Autodesk Inventor part; units mm, degrees
ref_plane "YZ Plane" through (0, 0, 0) normal (1, 0, 0) x (0, 1, 0)
ref_plane "XZ Plane" through (0, 0, 0) normal (0, 1, 0) x (-1, 0, 0)
ref_plane "XY Plane" through (0, 0, 0) normal (0, 0, 1) x (1, 0, 0)
sketch "Sketch1" plane through (0, 0, 0) normal (0, 0, 1) x (1, 0, 0)
  line L0 (-29.75, -11.25) -> (29.75, -11.25)
  line L1 (29.75, -11.25) -> (29.75, 11.25)
  line L2 (29.75, 11.25) -> (-29.75, 11.25)
  line L3 (-29.75, 11.25) -> (-29.75, -11.25)
  line L4 (-29.75, -11.25) -> (29.75, 11.25) construction
  line L5 (29.75, -11.25) -> (-29.75, 11.25) construction
  point P0 (0, 0)
  dimension "d0" = 59.5
  dimension "d1" = 22.5
extrude "Extrusion1" add sketch "Sketch1" against normal blind 1.6
fillet "Fillet1" radius 1.5 4 edges at (29.75, 11.25, -0.8) (29.75, -11.25, -0.8) (-29.75, 11.25, -0.8) (-29.75, -11.25, -0.8)
sketch "Sketch2" plane through (0, 0, 0) normal (0, 0, 1) x (1, 0, 0)
  circle A0 centre (-2.949, 1.26) radius 4.75
  line L0 (-28.25, -11.25) -> (28.25, -11.25)
  line L1 (-29.75, 9.75) -> (-29.75, -9.75)
  line L2 (-24.199, -4.44) -> (-19.799, -4.44)
  line L3 (-19.799, -4.44) -> (-19.799, -2.04)
  line L4 (-19.799, -2.04) -> (-24.199, -2.04)
  line L5 (-24.199, -2.04) -> (-24.199, -4.44)
  line L6 (-24.199, -4.44) -> (-19.799, -2.04) construction
  line L7 (-19.799, -4.44) -> (-24.199, -2.04) construction
  point P0 (0, 0)
  point P1 (-28.349, -5.24)
  point P2 (-21.999, -3.24)
  dimension "d5" = 9.5
  dimension "d15" = 12.51
  dimension "d16" = 26.801
  dimension "d17" = 6.01
  dimension "d18" = 1.401
  dimension "d19" = 4.4
  dimension "d20" = 2.4
  dimension "d21" = 6.35
  dimension "d22" = 2
extrude "Extrusion2" cut sketch "Sketch2" against normal through all
sketch "Sketch4" plane through (0, 0, 0) normal (0, 0, 1) x (1, 0, 0)
  line L0 (-28.25, -11.25) -> (28.25, -11.25)
  line L1 (-29.75, 9.75) -> (-29.75, -9.75)
  line L2 (6.731, -5.34) -> (22.931, -5.34)
  line L3 (22.931, -5.34) -> (22.931, 2.86)
  line L4 (22.931, 2.86) -> (6.731, 2.86)
  line L5 (6.731, 2.86) -> (6.731, -5.34)
  line L6 (6.731, -5.34) -> (22.931, 2.86) construction
  line L7 (22.931, -5.34) -> (6.731, 2.86) construction
  point P0 (0, 0)
  point P1 (-28.349, -5.24)
  point P2 (14.831, -1.24)
  dimension "d23" = 6.01
  dimension "d24" = 1.401
  dimension "d25" = 16.2
  dimension "d26" = 8.2
  dimension "d28" = 43.18
  dimension "d29" = 0.1
extrude "Extrusion4" cut sketch "Sketch4" against normal through all
sketch "Sketch5" plane through (0, 0, -1.6) normal (0, 0, -1) x (-1, 0, 0)
  line L0 (-29.75, 11.25) -> (29.75, 11.25) construction
  line L1 (29.75, 11.25) -> (29.75, -11.2327) construction
  line L2 (29.75, -11.2327) -> (-29.75, -11.2327) construction
  line L3 (-29.75, -11.2327) -> (-29.75, 11.25) construction
  line L4 (28.25, 11.25) -> (-28.25, 11.25)
  line L5 (-29.75, 9.75) -> (-29.75, -9.75)
  line L6 (29.75, -9.75) -> (29.75, 9.75)
  point P0 (0, 0)
decal "Decal1"
properties part number "rearPlate_PP"
The model under review builds one solid part; all positions refer to its coordinate system, in mm. A direction names the side the tool comes from. Round coordinates to 2 decimals unless told otherwise and drop trailing zeros. Loops run counter-clockwise (first coordinate to the right, second up) from the corner with the lowest first, then second, coordinate; pieces in that order, holes last. Notation, with made-up numbers: (60.5, 27) -> (69.5, 27) arc R28 cw to (69.5, 52) -> close; hole circle Ø9 at (-10.5, 5). An arc over 180 degrees is marked (long way). Answer as a JSON object with one key per item and string values. Group by question number.
1) We need section B-B on x = 20.5. Write out the cut boundary in (y, z), then the cut area to 3 significant figures.
2) We need section D-D on x = -4. Write out the cut boundary in (y, z), then the cut area to 3 significant figures.
3) For pin 1 Ø5.5 at (x, y) = (-2.949, 1.26) entering from +Z, flat-tipped, find the tip position at first contact; note if it passes through.
4) We need section A-A on y = 1.26. Write out the cut boundary in (x, z).
5) We need section C-C on z = -1.1. Write out the cut boundary in (x, y), then the cut area to 3 significant figures.
6) For line 1 (Y direction, x = 19.5, z = -1.05); line 2 (X direction, y = -0.5, z = -0.35); line 3 (X direction, y = 2.75, z = -0.65), list the stretches that pass through material, from the lowest coordinate up. Write a range as [from, to].
7) Mouldability with a two-part tool opening along Y and no side actions: class faces 1 (the face through (-22, -4.44, -1)), 2 (the face through (-29.3, -10.82, -0.81)), 3 (the face through (0, -5, -1.6)) as released by +Y, released by -Y, zero draft, split by the parting line, or undercut.
8) For faces 4 (the face through (-29.75, 0, -1)), 5 (the face through (6.731, -1, -1)), list the 3-axis set-ups (+Z, -Z, +X, -X, +Y, -Y) from which the entire face can be reached by the end or side of a thin tool; tool diameter is ignored.
Result set:
{
 "1": {"outline": "(-11.25, -1.6) -> (-5.34, -1.6) -> (-5.34, 0) -> (-11.25, 0) -> close; (2.86, -1.6) -> (11.25, -1.6) -> (11.25, 0) -> (2.86, 0) -> close", "area": "22.9 mm²"},
 "2": {"outline": "(-11.25, -1.6) -> (-3.37, -1.6) -> (-3.37, 0) -> (-11.25, 0) -> close; (5.89, -1.6) -> (11.25, -1.6) -> (11.25, 0) -> (5.89, 0) -> close", "area": "21.2 mm²"},
 "3": {"pin 1": "through"},
 "4": {"outline": "(-29.75, -1.6) -> (-7.7, -1.6) -> (-7.7, 0) -> (-29.75, 0) -> close; (1.8, -1.6) -> (6.73, -1.6) -> (6.73, 0) -> (1.8, 0) -> close; (22.93, -1.6) -> (29.75, -1.6) -> (29.75, 0) -> (22.93, 0) -> close"},
 "5": {"outline": "(-29.75, -9.75) arc R1.5 ccw to (-28.25, -11.25) -> (28.25, -11.25) arc R1.5 ccw to (29.75, -9.75) -> (29.75, 9.75) arc R1.5 ccw to (28.25, 11.25) -> (-28.25, 11.25) arc R1.5 ccw to (-29.75, 9.75) -> close; hole (-24.2, -4.44) -> (-19.8, -4.44) -> (-19.8, -2.04) -> (-24.2, -2.04) -> close; hole circle Ø9.5 at (-2.95, 1.26); hole (6.73, -5.34) -> (22.93, -5.34) -> (22.93, 2.86) -> (6.73, 2.86) -> close", "area": "1,120 mm²"},
 "6": {"line 1": "[-11.25, -5.34], [2.86, 11.25]", "line 2": "[-29.75, -7.36], [1.46, 6.73], [22.93, 29.75]", "line 3": "[-29.75, -7.46], [1.56, 6.73], [22.93, 29.75]"},
 "7": {"face 1": "undercut", "face 2": "released by -Y", "face 3": "zero draft"},
 "8": {"face 4": "+Z, -Z, -X, +Y, -Y", "face 5": "+Z, -Z"}
}
